from build123d import *

# Parameters (mm, degrees)
SKETCH1_W           = 30
SKETCH1_H           = 3
SKETCH1_W_2         = 3
SKETCH1_H_2         = 30
BOSS_EXTRUDE1_DEPTH = 3
SKETCH2_W           = 30
SKETCH2_H           = 3
CUT_EXTRUDE1_DEPTH  = 10


with BuildPart() as part:
    # Sketch1 → Boss-Extrude1 (new body)
    with BuildSketch(Plane(origin=(0, 0, 0), x_dir=(1, 0, 0), z_dir=(0, 1, 0))):
        with Locations((0, -56)):
            Rectangle(SKETCH1_W, SKETCH1_H)
        with Locations((-56, 0)):
            Rectangle(SKETCH1_W_2, SKETCH1_H_2)
        with Locations((0, 56)):
            Rectangle(SKETCH1_W, SKETCH1_H)
        Polygon((-54.5, -54.5), (-54.5, -15), (-54.5, 15), (-54.5, 54.5), (-15, 54.5), (15, 54.5), (54.5, 54.5), (54.5, 15), (54.5, -15), (54.5, -54.5), (15, -54.5), (-15, -54.5), align=None)
        with Locations((56, 0)):
            Rectangle(SKETCH1_W_2, SKETCH1_H_2)
    extrude(amount=BOSS_EXTRUDE1_DEPTH)

    # Sketch2 → Cut-Extrude1 (cut)
    with BuildSketch(Plane(origin=(0, 3, 0), x_dir=(1, 0, 0), z_dir=(0, 1, 0))):
        with Locations((0, -29)):
            Rectangle(SKETCH2_W, SKETCH2_H)
    extrude(amount=-CUT_EXTRUDE1_DEPTH, mode=Mode.SUBTRACT)


solid = part.part
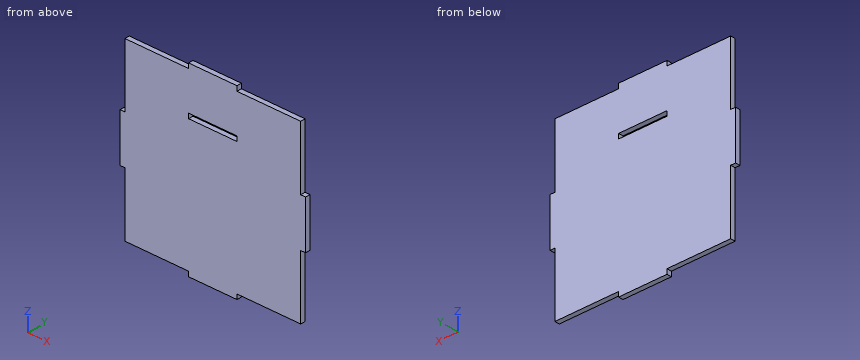
Model file for the job. Use its own axes, mm. Give positions to 0.01 mm unless a question says otherwise; leave off trailing zeros. Loops run counter-clockwise (first coordinate to the right, second up) from the corner with the lowest first, then second, coordinate; pieces in that order, holes last.
Item 1: Slice it at D-D (x = 19.5). Write the cut outline in (y, z), plus the area to 3 significant figures.
Check values:
outline: (0, -54.5) - (3, -54.5) - (3, 54.5) - (0, 54.5) - close
area: 327 mm2
Item 2: Drop flat-ended pins along their axis: P1, Ø1.5, axis at y = 1.5, z = 35, coming from the -X side; P2, Ø1.5, axis at x = -31.5, y = 2, coming from the -Z side; P3, Ø0.9, axis at y = 1, z = 56, coming from the +X side. Give the stop position or say it passes through.
Check values:
P1: stops at x = -54.5
P2: stops at z = -54.5
P3: stops at x = 15
Item 3: Slice it at B-B (y = 0.7). Write the cut outline in (x, z).
Check values:
outline: (-57.5, -15) - (-54.5, -15) - (-54.5, -54.5) - (-15, -54.5) - (-15, -57.5) - (15, -57.5) - (15, -54.5) - (54.5, -54.5) - (54.5, -15) - (57.5, -15) - (57.5, 15) - (54.5, 15) - (54.5, 54.5) - (15, 54.5) - (15, 57.5) - (-15, 57.5) - (-15, 54.5) - (-54.5, 54.5) - (-54.5, 15) - (-57.5, 15) - close; hole (-15, 27.5) - (15, 27.5) - (15, 30.5) - (-15, 30.5) - close
Item 4: Slice it at C-C (z = 32). Write the cut outline in (x, y).
Check values:
outline: (-54.5, 0) - (54.5, 0) - (54.5, 3) - (-54.5, 3) - close
Item 5: Drill centre lines: line 1 along Z through (x, y) = (-14, 1.7); line 2 along X through (y, z) = (0.3, 16). Where is each one in solid material? Low to high.
Check values:
line 1: z = -57.5 to 27.5, 30.5 to 57.5
line 2: x = -54.5 to 54.5
Item 6: Slice it at A-A (x = -12). Write the cut outline in (y, z).
Check values:
outline: (0, -57.5) - (3, -57.5) - (3, 27.5) - (0, 27.5) - close; (0, 30.5) - (3, 30.5) - (3, 57.5) - (0, 57.5) - close
